Model file for the job. Use its own axes, mm. A direction names the side the tool comes from. Give positions to 0.01 mm unless a question says otherwise; leave off trailing zeros. Loops run counter-clockwise (first coordinate to the right, second up) from the corner with the lowest first, then second, coordinate; pieces in that order, holes last. Notation, with made-up numbers: (58.5, -4.75) - (79.5, -4.75) arc R30 cw to (79.5, 28.25) - close; hole circle Ø2 at (8.25, 38). An arc over 180 degrees is marked (long way). Use a Markdown table: item, result.
Autodesk Inventor part; units mm, degrees
ref_plane "YZ Plane" through (0, 0, 0) normal (1, 0, 0) x (0, 1, 0)
ref_plane "XZ Plane" through (0, 0, 0) normal (0, 1, 0) x (-1, 0, 0)
ref_plane "XY Plane" through (0, 0, 0) normal (0, 0, 1) x (1, 0, 0)
sketch "スケッチ1" plane through (0, 0, 0) normal (0, 0, 1) x (1, 0, 0)
  line L0 (-31.5, 11.5) -> (31.5, 11.5)
  line L1 (31.5, 11.5) -> (31.5, -11.5)
  line L2 (31.5, -11.5) -> (-31.5, -11.5)
  line L3 (-31.5, -11.5) -> (-31.5, 11.5)
  line L4 (-31.5, 11.5) -> (31.5, -11.5) construction
  line L5 (31.5, 11.5) -> (-31.5, -11.5) construction
  line L6 (-30, 10) -> (30, 10) construction
  line L7 (30, 10) -> (30, -10) construction
  line L8 (30, -10) -> (-30, -10) construction
  line L9 (-30, -10) -> (-30, 10) construction
  line L10 (-30, 10) -> (30, -10) construction
  line L11 (30, 10) -> (-30, -10) construction
  circle A0 centre (-28, 8) radius 0.8
  line L12 (-31.5, 0) -> (31.5, 0) construction
  line L13 (0, 11.5) -> (0, -11.5) construction
  circle A1 centre (-28, -8) radius 0.8
  circle A2 centre (28, 8) radius 0.8
  circle A3 centre (28, -8) radius 0.8
  line L14 (-30.25, 10.25) -> (30.25, 10.25)
  line L15 (30.25, 10.25) -> (30.25, -10.25)
  line L16 (30.25, -10.25) -> (-30.25, -10.25)
  line L17 (-30.25, -10.25) -> (-30.25, 10.25)
  line L18 (-30.25, 10.25) -> (30.25, -10.25) construction
  line L19 (30.25, 10.25) -> (-30.25, -10.25) construction
  line L20 (-20, 10.25) -> (-20, -10.25)
  line L21 (20, 10.25) -> (20, -10.25)
  point P0 (0, 0)
  point P1 (0, 0)
  point P2 (20, -10.25)
  dimension "d0" = 63
  dimension "d1" = 60
  dimension "d2" = 20
  dimension "d3" = 23
  dimension "d4" = 1.6
  dimension "d5" = 2
  dimension "d6" = 2
  dimension "d7" = 20.5
  dimension "d8" = 60.5
  dimension "d13" = 10
extrude "押し出し1" add sketch "スケッチ1" against normal blind 1 contours L0 L1 L2 L3 | L14 L20 L16 L17 | L14 L21 L16 L20 | L14 L15 L16 L21
extrude "押し出し2" add sketch "スケッチ1" along normal blind 5 contours L0 L1 L2 L3
extrude "押し出し3" add sketch "スケッチ1" along normal blind 3.4 contours L14 L20 L16 L17 | L14 L15 L16 L21
fillet "フィレット1" radius 1 8 edges at (-31.5, -11.5, 2) (-31.5, 11.5, 2) (-20, 10.25, 1.7) (-20, -10.25, 1.7) (20, -10.25, 1.7) (20, 10.25, 1.7) (31.5, -11.5, 2) (31.5, 11.5, 2)
equation "\"d6\" = d5"
properties part number "StartStopSwitch_cover_01" material "アセタール樹脂、黒"
(1) Drill centre lines: probe 1 along Y at (x, z) = (-28, 0.3); probe 2 along X at (y, z) = (5.5, 0.75); probe 3 along Y at (x, z) = (-18, 4.15). Where is each one in solid material? Low to high. Write a range as [from, to].
Computed:
| item | result |
|---|---|
| probe 1 | [-11.5, -8.8], [-7.2, 7.2], [8.8, 11.5] |
| probe 2 | [-31.5, -20], [20, 31.5] |
| probe 3 | [-11.5, -10.25], [10.25, 11.5] |
(2) Slice it at C-C, the plane y = 8. Write the cut outline in (x, z), plus the area to 3 significant figures.
Computed:
| item | result |
|---|---|
| outline | (-31.5, -1) - (-28.8, -1) - (-28.8, 3.4) - (-30.25, 3.4) - (-30.25, 5) - (-31.5, 5) - close; (-27.2, -1) - (27.2, -1) - (27.2, 3.4) - (20, 3.4) - (20, 0) - (-20, 0) - (-20, 3.4) - (-27.2, 3.4) - close; (28.8, -1) - (31.5, -1) - (31.5, 5) - (30.25, 5) - (30.25, 3.4) - (28.8, 3.4) - close |
| area | 131 mm² |
(3) 3-axis set-ups, long thin cutter, end or side, ignore diameter. For faces 1 (the flat face through (-31.5, 0, 2)), 2 (the flat face through (30.25, 0, 4)): which of +Z, -Z, +X, -X, +Y, -Y reach the whole face in a straight line?
Computed:
| item | result |
|---|---|
| face 1 | +Z, -Z, -X, +Y, -Y |
| face 2 | +Z |
(4) Mould opens along X. For faces 3 (the flat face through (0, -10.25, 3)), 4 (the flat face through (0, 0, -1)), 5 (the flat face through (31.5, 0, 2)) say: pulls with the +X half, pulls with the -X half, needs draft (parallel to the pull), parting line crosses it, or undercut.
Computed:
| item | result |
|---|---|
| face 3 | undercut |
| face 4 | needs draft |
| face 5 | pulls with the +X half |
(5) Pin check, flat tips, straight feed: P1, Ø3.5, axis at x = -25.5, y = 2.5, coming from the +Z side; P2, Ø2, axis at x = 2.5, y = -6.5, coming from the +Z side. Stop position of each tip, or through.
Computed:
| item | result |
|---|---|
| P1 | z = 3.4 |
| P2 | z = 0 |
(6) Slice it at B-B, the plane z = 2.45. Write the cut outline in (x, y).
Computed:
| item | result |
|---|---|
| outline | (-31.5, -10.5) arc R1 ccw to (-30.5, -11.5) - (30.5, -11.5) arc R1 ccw to (31.5, -10.5) - (31.5, 10.5) arc R1 ccw to (30.5, 11.5) - (-30.5, 11.5) arc R1 ccw to (-31.5, 10.5) - close; hole circle Ø1.6 at (-28, -8); hole circle Ø1.6 at (-28, 8); hole (-20, -9.25) arc R1 ccw to (-19, -10.25) - (19, -10.25) arc R1 ccw to (20, -9.25) - (20, 9.25) arc R1 ccw to (19, 10.25) - (-19, 10.25) arc R1 ccw to (-20, 9.25) - close; hole circle Ø1.6 at (28, -8); hole circle Ø1.6 at (28, 8) |
(7) Slice it at A-A, the plane x = -28. Write the cut outline in (y, z), plus the area to 3 significant figures.
Computed:
| item | result |
|---|---|
| outline | (-11.5, -1) - (-8.8, -1) - (-8.8, 3.4) - (-10.25, 3.4) - (-10.25, 5) - (-11.5, 5) - close; (-7.2, -1) - (7.2, -1) - (7.2, 3.4) - (-7.2, 3.4) - close; (8.8, -1) - (11.5, -1) - (11.5, 5) - (10.25, 5) - (10.25, 3.4) - (8.8, 3.4) - close |
| area | 91.1 mm² |
(8) Slice it at D-D, the plane x = 26. Write the cut outline in (y, z).
Computed:
| item | result |
|---|---|
| outline | (-11.5, -1) - (11.5, -1) - (11.5, 5) - (10.25, 5) - (10.25, 3.4) - (-10.25, 3.4) - (-10.25, 5) - (-11.5, 5) - close |
